Input: part model. Units: mm. Frame: model coordinates. Face numbers are marked on the shaded views. A direction names the side the tool comes from. Round coordinates to 2 decimals unless told otherwise and drop trailing zeros. Order: outer loops, then holes, each group sorted by start corner. A loop starts at its lowest first (then second) coordinate and runs counter-clockwise, first axis right, second up. Notation, with made-up numbers: (65, 56.25) -> (119, 56.25) arc R28 ccw to (119, 92.25) -> close; hole circle Ø4 at (77, 89). An arc over 180 degrees is marked (long way). Use a Markdown table: item, result.
from build123d import *

# Parameters (mm, degrees)
F1_DEPTH = 7.62
F2_R     = 10.1865714181
F3_DEPTH = 6.35
F5_R     = 7.316904296
F6_DEPTH = 6.35
F9_R     = 2.5656803157


# Not quite as in the source:
# - a fillet or chamfer that OpenCascade refuses, or shapes differently, is made with other operations: its cross-section is extruded or revolved along the edge and cut away or added


with BuildPart() as f1:
    # F0 (on Top) → F1 (new body)
    with BuildSketch(Plane.XY):
        Polygon((7.62, -13.1982271537), (15.24, 0), (7.62, 13.1982271537), (-7.62, 13.1982271537), (-15.24, 0), (-7.62, -13.1982271537), align=None)
    extrude(amount=F1_DEPTH)

    # F2 (on face) → F3 (join)
    with BuildSketch(Plane.XY.offset(7.62)):
        Circle(F2_R)
    extrude(amount=F3_DEPTH)

    # F4: fillet of radius 7.62 on 1 edges, made by hand

    # F4_s1 → F4_t2 (revolve, cut)
    with BuildSketch(Plane.XZ):
        with BuildLine():
            ThreePointArc((10.1865714181, 7.62), (7.5918389432, 12.1698711326), (2.6731500935, 13.97))
            Line((2.6731500935, 13.97), (10.1865714181, 13.97))
            Line((10.1865714181, 13.97), (10.1865714181, 7.62))
        make_face()
    revolve(axis=Axis((0, 0, 13.97), (0, 0, 1)), mode=Mode.SUBTRACT)

    # F5 (on face) → F6 (cut, through all)
    with BuildSketch(Plane.XY.offset(13.97)):
        Circle(F5_R)
    extrude(amount=-F6_DEPTH, mode=Mode.SUBTRACT)

    # F7 (on Front) → F8 (revolve, cut)
    with BuildSketch(Plane.XZ):
        with BuildLine():
            Line((7.2382027283, 7.666405756), (9.4514777884, 7.6440493576))
            ThreePointArc((9.4514777884, 7.6440493576), (8.7401460246, 9.8436861794), (7.2382027283, 11.6011165082))
            Line((7.2382027283, 11.6011165082), (7.2382027283, 7.666405756))
        make_face()
    revolve(axis=Axis((0, 0, 13.97), (0, 0, 1)), mode=Mode.SUBTRACT)

    # F9 (on face) → F10 (revolve, cut)
    with BuildSketch(Plane.XZ.offset(13.1982271537)):
        with Locations((-2.5616665371, 3.7216017954)):
            Circle(F9_R)
    revolve(axis=Axis((-7.62, -13.1982271537, 3.81), (0, 0, -1)), mode=Mode.SUBTRACT)


solid = f1.part
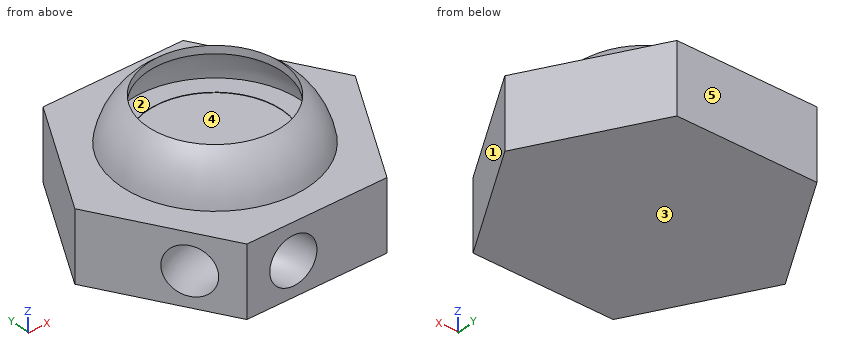
1) Line query: L1, parallel to Z at x = -9, y = -5; L2, parallel to Y at x = 7, z = 11; L3, parallel to X at y = 7.5, z = 8.75. Output: solid intervals per line, ascending. Write a range as [from, to].
Results found:
| item | result |
|---|---|
| L1 | z = [0, 7.62] |
| L2 | y = [-5.18, -3.65], [3.65, 5.18] |
| L3 | x = [-6.47, -5.35], [5.35, 6.47] |
2) Set-up query: the marked faces 4 and 5. Return all of +Z, -Z, +X, -X, +Y, -Y with unobstructed straight access to the full face (end or side cutting, diameter ignored); none if empty.
Results found:
| item | result |
|---|---|
| face 4 | +Z |
| face 5 | +Z, -Z, +X, -X, +Y |
3) Pin query (flat end, axial travel): pin 1 Ø1 at (x, y) = (-6, -2.5) entering from +Z; pin 2 Ø2 at (y, z) = (6, 4) entering from +X; pin 3 Ø3 at (x, z) = (-8.5, 10) entering from -Y. Return the tip coordinate at first contact, or that it passes through.
Results found:
| item | result |
|---|---|
| pin 1 | stops at z = 7.62 |
| pin 2 | stops at x = 12.35 |
| pin 3 | stops at y = -6.53 |
4) Pull-direction query (Z, two-part tool) for the marked faces 1, 2 and 3; classes: +Z half, -Z half, draft (parallel to the pull), parting line (faces both ways), or undercut.
Results found:
| item | result |
|---|---|
| face 1 | draft |
| face 2 | undercut |
| face 3 | -Z half |
5) Cut plane B-B on z = 4.5. Return loops of the section in (x, y).
Results found:
| item | result |
|---|---|
| outline | (-15.24, 0) -> (-11.37, -6.7) arc R7.5 cw to (-0.12, -13.2) -> (7.62, -13.2) -> (15.24, 0) -> (7.62, 13.2) -> (-7.62, 13.2) -> close; (-8.93, -10.93) -> (-7.62, -13.2) -> (-5.01, -13.2) arc R2.61 ccw to start |
6) Cut plane A-A on z = 7. Return loops of the section in (x, y), and give its area (3 significant figures).
Results found:
| item | result |
|---|---|
| outline | (-15.24, 0) -> (-7.62, -13.2) -> (7.62, -13.2) -> (15.24, 0) -> (7.62, 13.2) -> (-7.62, 13.2) -> close |
| area | 603 mm² |
7) Cut plane C-C on y = 10.75. Return loops of the section in (x, z), and give its area (3 significant figures).
Results found:
| item | result |
|---|---|
| outline | (-9.03, 0) -> (9.03, 0) -> (9.03, 7.62) -> (-9.03, 7.62) -> close |
| area | 138 mm² |
